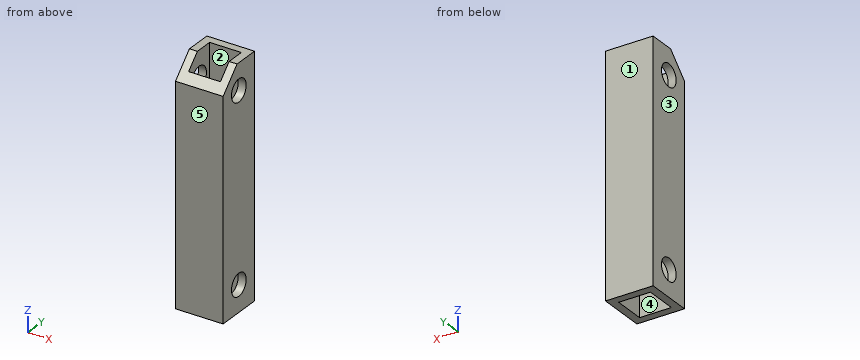
```python
from build123d import *

# Parameters (mm, degrees)
SKETCH_1_W          = 9
SKETCH_1_H          = 9
SKETCH_1_W_2        = 6
SKETCH_1_H_2        = 6
EXTRUDE_1_DEPTH     = 45
SKETCH_2_R          = 2.1
CUT_EXTRUDE_1_DEPTH = 30
CUT_EXTRUDE_3_DEPTH = 10


with BuildPart() as part:
    # ｽｹｯﾁ1 → ﾎﾞｽ - 押し出し1 (new body)
    with BuildSketch(Plane.XY):
        Rectangle(SKETCH_1_W, SKETCH_1_H)
        Rectangle(SKETCH_1_W_2, SKETCH_1_H_2, mode=Mode.SUBTRACT)
    extrude(amount=EXTRUDE_1_DEPTH)

    # ｽｹｯﾁ2 → ｶｯﾄ - 押し出し1 (cut)
    with BuildSketch(Plane(origin=(4.5, 0, 0), x_dir=(0, 0, -1), z_dir=(1, 0, 0))):
        with Locations((-40, 0)):
            Circle(SKETCH_2_R)
        with Locations((-5, 0)):
            Circle(SKETCH_2_R)
    extrude(amount=-CUT_EXTRUDE_1_DEPTH, mode=Mode.SUBTRACT)

    # ｽｹｯﾁ3 → ｶｯﾄ - 押し出し3 (cut)
    with BuildSketch(Plane(origin=(4.5, 0, 0), x_dir=(0, 0, -1), z_dir=(1, 0, 0))):
        Polygon((-45, -4.5), (-45, -0.5), (-41, -4.5), align=None)
    extrude(amount=-CUT_EXTRUDE_3_DEPTH, mode=Mode.SUBTRACT)


solid = part.part
```
Input: part model. Units: mm. Frame: model coordinates. Face numbers are marked on the shaded views. A direction names the side the tool comes from. Round coordinates to 2 decimals unless told otherwise and drop trailing zeros. Loops run counter-clockwise (first coordinate to the right, second up) from the corner with the lowest first, then second, coordinate; pieces in that order, holes last.
1) Section query C-C on x = 1.75. Return the cut outline in (y, z), plus the area to 3 significant figures.
Ans:
outline: (-4.5, 0) - (-3, 0) - (-3, 42.5) - (-4.5, 41) - close; (3, 0) - (4.5, 0) - (4.5, 45) - (3, 45) - close
area: 130 mm2
2) Section query B-B on y = 0. Return the cut outline in (x, z), plus the area to 3 significant figures.
Ans:
outline: (-4.5, 0) - (-3, 0) - (-3, 2.9) - (-4.5, 2.9) - close; (-4.5, 7.1) - (-3, 7.1) - (-3, 37.9) - (-4.5, 37.9) - close; (-4.5, 42.1) - (-3, 42.1) - (-3, 45) - (-4.5, 45) - close; (3, 0) - (4.5, 0) - (4.5, 2.9) - (3, 2.9) - close; (3, 7.1) - (4.5, 7.1) - (4.5, 37.9) - (3, 37.9) - close; (3, 42.1) - (4.5, 42.1) - (4.5, 45) - (3, 45) - close
area: 110 mm2
3) Pin query (flat end, axial travel): pin 1 (2.5 mm diameter, centred on y = 0, z = 5, fed in from +X). Return the tip coordinate at first contact, or that it passes through.
Ans:
pin 1: passes through
4) Set-up query: the marked faces 4 and 5. Return all of +Z, -Z, +X, -X, +Y, -Y with unobstructed straight access to the full face (end or side cutting, diameter ignored); none if empty.
Ans:
face 4: +Z, -Z
face 5: +Z, -Z, +X, -X, -Y
5) Section query D-D on x = -3.5. Return the cut outline in (y, z).
Ans:
outline: (-4.5, 0) - (4.5, 0) - (4.5, 45) - (-0.5, 45) - (-4.5, 41) - close; hole circle Ø4.2 at (0, 5); hole circle Ø4.2 at (0, 40)
6) Pull-direction query (X, two-part tool) for the marked faces 1, 2 and 3; classes: released by +X, released by -X, zero draft, split by the parting line, or undercut.
Ans:
face 1: zero draft
face 2: undercut
face 3: released by -X
7) Material intervals for line 1 (X direction, y = -2, z = 11.5); line 2 (Y direction, x = 4.1, z = 40), sorted ascending.
Ans:
line 1: x = -4.5 to -3, 3 to 4.5
line 2: y = -4.5 to -2.1, 2.1 to 4.5
8) Section query A-A on z = 40. Return the cut outline in (x, y).
Ans:
outline: (-4.5, -4.5) - (4.5, -4.5) - (4.5, -2.1) - (3, -2.1) - (3, -3) - (-3, -3) - (-3, -2.1) - (-4.5, -2.1) - close; (-4.5, 2.1) - (-3, 2.1) - (-3, 3) - (3, 3) - (3, 2.1) - (4.5, 2.1) - (4.5, 4.5) - (-4.5, 4.5) - close
